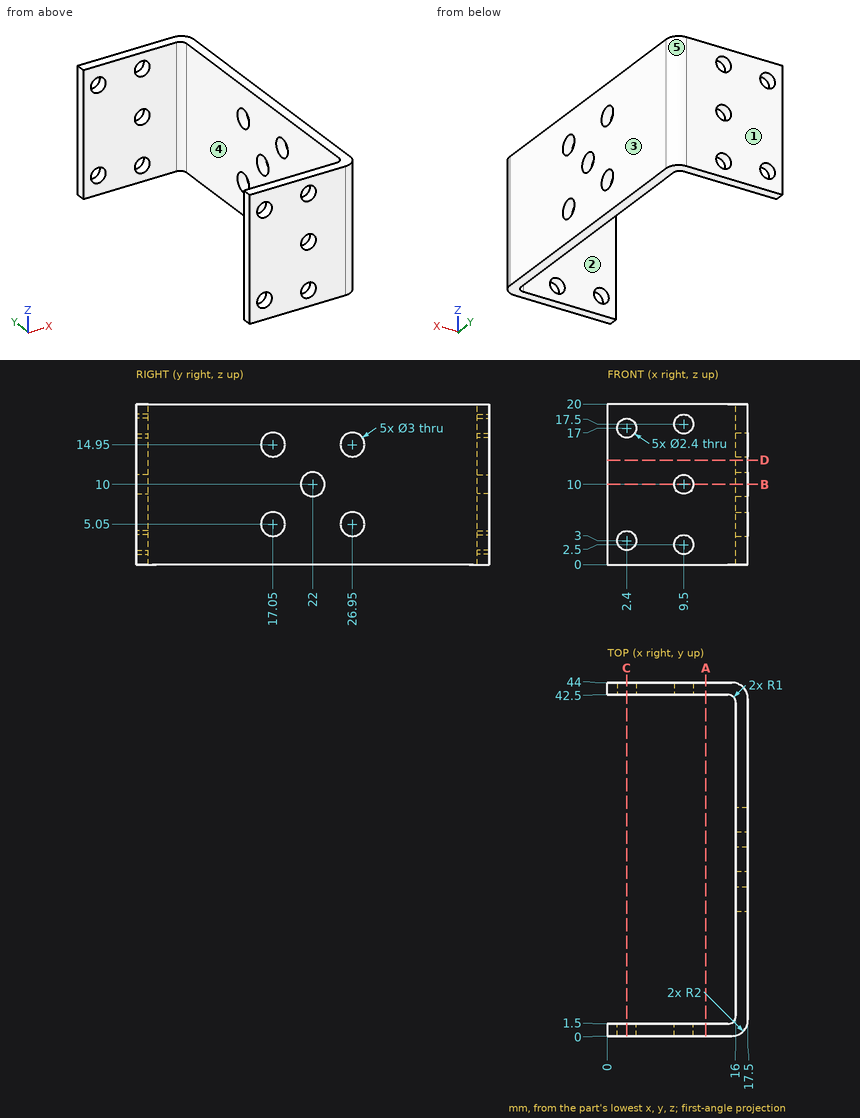
Design review of the part shown in the three views and the two pictorial views. Dimensions are in mm from the part's minimum x, y and z. A direction names the side the tool comes from. Coordinates: 2 decimals unless noted, no trailing zeros. Loops run counter-clockwise (first coordinate to the right, second up) from the corner with the lowest first, then second, coordinate; pieces in that order, holes last.
Q1. To check wall thickness, follow line 1 (Y direction, x = 13.25, z = 12.5); line 2 (X direction, y = 0.7, z = 2.5); line 3 (X direction, y = 43.6, z = 17.5). State the ranges of each line that lie inside material, in increasing order.
Reported:
line 1: y = 0 to 1.5, 42.5 to 44
line 2: x = 0 to 1.31, 3.49 to 8.3, 10.7 to 17.02
line 3: x = 0 to 1.31, 3.49 to 8.3, 10.7 to 16.7
Q2. We need section A-A on x = 12.25. State the section outline as (y, z) points.
Reported:
outline: (0, 0) - (1.5, 0) - (1.5, 20) - (0, 20) - close; (42.5, 0) - (44, 0) - (44, 20) - (42.5, 20) - close
Q3. We need section C-C on x = 2.4. State the section outline as (y, z) points.
Reported:
outline: (0, 0) - (1.5, 0) - (1.5, 1.8) - (0, 1.8) - close; (0, 4.2) - (1.5, 4.2) - (1.5, 15.8) - (0, 15.8) - close; (0, 18.2) - (1.5, 18.2) - (1.5, 20) - (0, 20) - close; (42.5, 0) - (44, 0) - (44, 1.8) - (42.5, 1.8) - close; (42.5, 4.2) - (44, 4.2) - (44, 15.8) - (42.5, 15.8) - close; (42.5, 18.2) - (44, 18.2) - (44, 20) - (42.5, 20) - close
Q4. We need section B-B on z = 10. State the section outline as (x, y) points.
Reported:
outline: (0, 0) - (8.3, 0) - (8.3, 1.5) - (0, 1.5) - close; (0, 42.5) - (8.3, 42.5) - (8.3, 44) - (0, 44) - close; (10.7, 0) - (15.5, 0) arc R2 ccw to (17.5, 2) - (17.5, 20.5) - (16, 20.5) - (16, 2.5) arc R1 cw to (15, 1.5) - (10.7, 1.5) - close; (10.7, 42.5) - (15, 42.5) arc R1 cw to (16, 41.5) - (16, 23.5) - (17.5, 23.5) - (17.5, 42) arc R2 ccw to (15.5, 44) - (10.7, 44) - close
Q5. For pin 1 (2.5 mm diameter, centred on y = 17.05, z = 5.05, fed in from -X); pin 2 (3.5 mm diameter, centred on y = 26.95, z = 14.95, fed in from -X), all flat-tipped, find the tip position at first contact; note any pin that passes through.
Reported:
pin 1: passes through
pin 2: stops at x = 16
Q6. Tool access review of the marked faces 4 and 5: name each direction out of +Z, -Z, +X, -X, +Y, -Y from which nothing blocks a thin tool from reaching the whole face with its end or side.
Reported:
face 4: +Z, -Z, -X
face 5: +Z, -Z, +X, +Y
Q7. The part is to be moulded in two halves that separate along Y. For the marked faces 1, 2 and 3, say which applies: +Y half, -Y half, draft (parallel to the pull), parting line (faces both ways), or undercut.
Reported:
face 1: +Y half
face 2: undercut
face 3: draft
Q8. We need section D-D on z = 13. State the section outline as (x, y) points.
Reported:
outline: (0, 0) - (15.5, 0) arc R2 ccw to (17.5, 2) - (17.5, 42) arc R2 ccw to (15.5, 44) - (0, 44) - (0, 42.5) - (15, 42.5) arc R1 cw to (16, 41.5) - (16, 2.5) arc R1 cw to (15, 1.5) - (0, 1.5) - close
